Design review of the part built by this model. Coordinates are the model's own, in mm. Face numbers are marked on the shaded views. A direction names the side the tool comes from. Coordinates: 2 decimals unless noted, no trailing zeros. Write each loop counter-clockwise with the first axis right and the second up, starting at its lowest first coordinate (ties: lowest second). Pieces come first, ordered by that corner, then holes.
Q1. Add section C-C, the plane x = -15.5. Give the boundary of the cut face in (y, z), plus the area to 3 significant figures.
Q2. Add section D-D, the plane y = 1.5. Give the boundary of the cut face in (x, z), plus the area to 3 significant figures.
Q3. The part is to be moulded in two halves that separate along X. For the marked faces 4 and 5, say which applies: +X half, -X half, draft (parallel to the pull), parting line (faces both ways), or undercut.
Q4. Clearance check with flat-ended pins moving along their axes: pin 1 Ø0.9 at (y, z) = (10.5, 2) entering from -X; pin 2 Ø1.5 at (y, z) = (-22, -37) entering from -X; pin 3 Ø5 at (x, y) = (-4, -102.5) entering from +Z. State where each tip first meets the part, or that it passes through.
Q5. Add section B-B, the plane y = 15.5. Give the boundary of the cut face in (x, z).
Q6. Machinability: for the marked faces 1, 2 and 3, which of the approach directions +Z, -Z, +X, -X, +Y, -Y give a long, thin tool a straight path to every point of the face, cutting with its end or side? Answer none if there is none.
Q7. To check wall thickness, follow probe 1 along X at (y, z) = (-116.2, -20); probe 2 along X at (y, z) = (-68.5, -9); probe 3 along Y at (x, z) = (-15, 2). State the ranges of each line that lie inside material, in increasing order.
Q8. Add section A-A, the plane z = -35. Give the boundary of the cut face in (x, y), plus the area to 3 significant figures.
Autodesk Inventor part; units mm, degrees
ref_plane "YZ Plane" through (0, 0, 0) normal (1, 0, 0) x (0, 1, 0)
ref_plane "XZ Plane" through (0, 0, 0) normal (0, 1, 0) x (-1, 0, 0)
ref_plane "XY Plane" through (0, 0, 0) normal (0, 0, 1) x (1, 0, 0)
sketch "Boceto1" plane through (0, 0, 0) normal (0, 0, 1) x (1, 0, 0)
  line L0 (-21, 21) -> (21, 21)
  line L1 (21, 21) -> (21, -21)
  line L2 (21, -21) -> (-21, -21)
  line L3 (-21, -21) -> (-21, 21)
  circle A0 centre (0, 0) radius 11.5
  circle A1 centre (-15.5, 15.5) radius 2.25
  circle A2 centre (-15.5, -15.5) radius 2.25
  circle A3 centre (15.5, -15.5) radius 2.25
  circle A4 centre (15.5, 15.5) radius 2.25
  dimension "d0" = 42
  dimension "d1" = 42
  dimension "d2" = 23
  dimension "d6" = 4.5
  dimension "d7" = 4.5
  dimension "d8" = 4.5
  dimension "d9" = 4.5
extrude "Extrusión1" add sketch "Boceto1" along normal blind 3
sketch "Boceto28" plane through (0, 0, 3) normal (0, 0, 1) x (1, 0, 0)
  line L0 (-21.25, -24) -> (21.25, -24)
  line L1 (21.25, -24) -> (21.25, -21)
  line L2 (-21.25, -21) -> (-21.25, -24)
  line L3 (-21, -21) -> (21, -21)
  line L4 (21.25, -21) -> (-21.25, -21)
  point P0 (0, 0)
extrude "Extrusión24" add sketch "Boceto28" against normal blind 43
sketch "Boceto29" plane through (-21.25, -21, -40) normal (0, 1, 0) x (1, 0, 0)
  line L0 (30.25, -12) -> (12.25, -12)
  line L1 (0, 0) -> (42.5, 0)
  line L2 (12.25, 0) -> (30.25, 0)
  line L3 (12.25, 0) -> (12.25, -12)
  line L4 (30.25, 0) -> (30.25, -12)
  point P0 (21.25, -40)
extrude "Extrusión25" cut sketch "Boceto29" against normal blind 3
sketch "Boceto33" plane through (21.25, -24, 3) normal (1, 0, 0) x (0, 0, -1)
  line L0 (43, 0) -> (33, 0)
  line L1 (33, 0) -> (33, 3)
  line L2 (43, 0) -> (46, 0)
  line L3 (46, 0) -> (46, 13)
  line L4 (46, 13) -> (43, 13)
  line L5 (43, 13) -> (33, 3)
  line L6 (0, 45) -> (0, 3)
  line L7 (0, 0) -> (43, 0)
  line L8 (0, 24) -> (0, 0)
  line L9 (0, 0) -> (24, 0)
  line L10 (24, 0) -> (24, 3)
  line L11 (0, 3) -> (43, 3)
  line L12 (0, 24) -> (3, 24)
  line L13 (3, 45) -> (3, 3)
  line L14 (3, 24) -> (24, 3)
  point P0 (0, 3)
  dimension "d153" = 10
  dimension "d154" = 3
  dimension "d155" = 13
  dimension "d156" = 3
  dimension "d181" = 24
extrude "Extrusión28" add sketch "Boceto33" along normal blind 3 contours L0 L1 L5 L4 L3 L2 | L7 L8 L11 L10 | L11 L13 L14 | L11 L6 L12 L13
sketch "Boceto34" plane through (-21.25, -24, 3) normal (-1, 0, 0) x (0, 0, 1)
  line L0 (-46, 0) -> (-46, 13)
  line L1 (-46, 13) -> (-43, 13)
  line L2 (-46, 13) -> (-43, 13)
  line L3 (-43, 13) -> (-33, 3)
  line L4 (-43, 0) -> (-46, 0)
  line L5 (-46, 13) -> (-46, 0)
  line L6 (-46, 0) -> (-33, 0)
  line L7 (-33, 3) -> (-33, 0)
  line L8 (-24, 0) -> (-24, 3)
  line L9 (-24, 3) -> (-3, 24)
  line L10 (0, 24) -> (-3, 24)
  line L11 (-24, 0) -> (0, 0)
  line L12 (0, 0) -> (0, 24)
extrude "Extrusión29" add sketch "Boceto34" along normal blind 3
sketch "Boceto36" plane through (0, 0, -40) normal (0, 0, -1) x (-1, 0, 0)
  line L0 (9, -21) -> (9, -24)
  line L1 (9, -24) -> (21.25, -24)
  line L2 (21.25, -24) -> (21.25, -11)
  line L3 (9, -21) -> (9, -24)
  line L4 (-9, -24) -> (-9, -21)
  line L5 (-9, -21) -> (-9, -24)
  line L6 (-21, -21) -> (-21, 21)
  line L7 (-21.25, -11) -> (-9, -21)
  line L8 (-21.25, -11) -> (-21.25, -24)
  line L9 (24.25, -24) -> (-24.25, -24)
  line L10 (-9, -24) -> (-21.25, -24)
  line L11 (9, -21) -> (21.25, -11)
extrude "Extrusión31" add sketch "Boceto36" along normal blind 3
sketch "Boceto37" plane through (-21, -21, 0) normal (0, 1, 0) x (1, 0, 0)
  line L0 (45.25, 40) -> (45.25, 30)
  line L1 (42.25, 21) -> (42.25, 0)
  line L2 (45.25, 30) -> (42.25, 30)
  line L3 (42.25, 30) -> (42.25, 21)
  line L4 (42.25, 21) -> (45.25, 21)
  line L5 (45.25, 21) -> (45.25, 30)
  line L6 (30, 40) -> (30, 43)
  line L7 (12, 43) -> (12, 28)
  line L8 (30, 40) -> (12, 40)
  line L9 (12, 40) -> (12, 43)
  line L10 (12, 43) -> (30, 43)
  line L11 (30, 43) -> (30, 40)
  line L12 (-0.25, 21) -> (-0.25, 30)
  line L13 (-3.25, 0) -> (-3.25, 21)
  line L14 (-0.25, 30) -> (-3.25, 30)
  line L15 (-3.25, 30) -> (-3.25, 21)
  line L16 (-3.25, 21) -> (-0.25, 21)
  line L17 (-0.25, 21) -> (-0.25, 30)
extrude "Extrusión32" add sketch "Boceto37" against normal blind 3
sketch "Boceto38" plane through (0, 0, 3) normal (0, 0, 1) x (1, 0, 0)
  line L0 (-21.25, 0) -> (-21.25, -21)
  line L1 (-21, -21) -> (-21.25, -21)
  line L2 (-21.25, 0) -> (-21, 0)
  line L3 (-21, 0) -> (-21, -21)
  line L4 (-21, -21) -> (-21.25, -21)
  line L5 (-21.25, -21) -> (-21.25, 0)
  line L6 (21, -21) -> (21, 21)
  line L7 (21.25, 0) -> (21.25, -21)
  line L8 (21, -21) -> (21.25, -21)
  line L9 (21.25, -21) -> (21.25, 0)
  line L10 (21.25, 0) -> (21, 0)
  line L11 (21, 0) -> (21, -21)
extrude "Extrusión33" add sketch "Boceto38" against normal blind 3
sketch "Boceto50" plane through (24.25, -24, -43) normal (0, -1, 0) x (1, 0, 0)
  line L0 (-45.5, 0) -> (-48.5, 0)
  line L1 (-48.5, 0) -> (-48.5, 46)
  line L2 (-48.5, 0) -> (-48.5, 46)
  line L3 (-48.5, 46) -> (-42.5, 46)
  line L4 (-42.5, 46) -> (-42.5, 3)
  line L5 (-48.5, 0) -> (0, 0)
  line L6 (-48.5, 0) -> (0, 0)
  line L7 (0, 0) -> (0, 46)
  line L8 (0, 46) -> (-6, 46)
  line L9 (-6, 46) -> (-6, 3)
  line L10 (-42.5, 3) -> (-6, 3)
  dimension "d183" = 6
  dimension "d184" = 6
extrude "Extrusión39" add sketch "Boceto50" along normal blind 94
sketch "Boceto51" plane through (24.25, -24, 3) normal (1, 0, 0) x (0, 0, -1)
  line L0 (18, -94) -> (28, -94)
  line L1 (28, -94) -> (28, -91)
  line L2 (28, -91) -> (18, -91)
  line L3 (18, -91) -> (18, -94)
  point P0 (3, 24)
  dimension "d171" = 10
  dimension "d172" = 3
extrude "Extrusión40" add sketch "Boceto51" along normal blind 10
sketch "Boceto52" plane through (-24.25, -24, 3) normal (-1, 0, 0) x (0, 0, 1)
  line L0 (0, -94) -> (-46, -94)
  line L1 (-18, -91) -> (-18, -94)
  line L2 (-23, -94) -> (-18, -94)
  line L3 (-18, -94) -> (-18, -91)
  line L4 (-28, -91) -> (-18, -91)
  line L5 (-18, -91) -> (-28, -91)
  line L6 (-28, -94) -> (-28, -91)
  line L7 (-28, -91) -> (-28, -94)
  line L8 (-28, -94) -> (-23, -94)
  point P0 (-3, 24)
extrude "Extrusión41" add sketch "Boceto52" along normal blind 10
sketch "Boceto56" plane through (-24.25, -115, -15) normal (0, 1, 0) x (1, 0, 0)
  line L0 (48.5, 0) -> (58.5, 0)
  line L1 (48.5, 10) -> (58.5, 10)
  line L2 (0, 10) -> (-10, 10)
  line L3 (0, 0) -> (-10, 0)
  line L4 (-10, 0) -> (-10, 10)
  circle A0 centre (-5, 5) radius 2
  circle A1 centre (53.5, 5) radius 2
  point P0 (24.25, -15)
  dimension "d185" = 4
  dimension "d186" = 4
extrude "Extrusión43" cut sketch "Boceto56" against normal blind 3
sketch "Boceto66" plane through (24.25, -24, 3) normal (1, 0, 0) x (0, 0, -1)
  line L0 (3, 24) -> (24, 3)
  circle A0 centre (23, -7) radius 1.6
  dimension "d224" = 3.2
extrude "Extrusión48" cut sketch "Boceto66" against normal blind 10
sketch "Boceto67" plane through (-24.25, -24, 3) normal (-1, 0, 0) x (0, 0, 1)
  line L0 (0, 24) -> (0, -94)
  circle A0 centre (-23, -7) radius 1.6
  point P0 (-3, 24)
  point P1 (-24, 3)
  dimension "d228" = 3.2
extrude "Extrusión50" cut sketch "Boceto67" against normal blind 10
properties part number "Torre Motor Definitiva Pont" material "Plástico ABS"
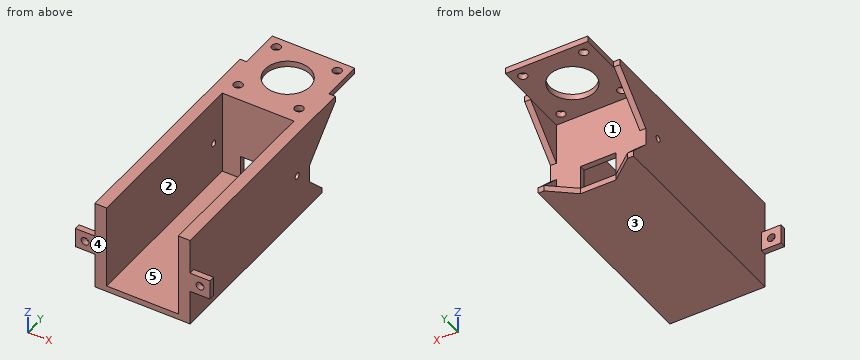
Here are the results:
1. outline: (-118, -43) - (-15.69, -43) - (-15.69, -40) - (-21, -40) - (-21, 0) - (-17.75, 0) - (-17.75, 3) - (-24, 3) - (-24, -40) - (-118, -40) - close; (-13.25, 0) - (13.25, 0) - (13.25, 3) - (-13.25, 3) - close; (17.75, 0) - (21, 0) - (21, 3) - (17.75, 3) - close
1. area: 535 mm2
2. outline: (-21, 0) - (-11.4, 0) - (-11.4, 3) - (-21, 3) - close; (11.4, 0) - (21, 0) - (21, 3) - (11.4, 3) - close
2. area: 57.6 mm2
3. face 4: draft
3. face 5: undercut
4. pin 1: stops at x = -21
4. pin 2: stops at x = -24.25
4. pin 3: stops at z = -40
5. outline: (-21, 0) - (-17.75, 0) - (-17.75, 3) - (-21, 3) - close; (-13.25, 0) - (13.25, 0) - (13.25, 3) - (-13.25, 3) - close; (17.75, 0) - (21, 0) - (21, 3) - (17.75, 3) - close
6. face 1: +Y
6. face 2: +Z, -Y
6. face 3: -Z, +X, -X, +Y, -Y
7. probe 1: x = -34.25 to -31.25, -27.25 to -18.25, 18.25 to 27.25, 31.25 to 34.25
7. probe 2: x = -24.25 to -18.25, 18.25 to 24.25
7. probe 3: y = -24 to -17.69, -13.31 to 13.31, 17.69 to 21
8. outline: (-24.25, -118) - (-18.25, -118) - (-18.25, -24) - (-9, -24) - (-9, -21) - (-21.25, -21) - (-21.25, -16) - (-24.25, -16) - close; (9, -24) - (18.25, -24) - (18.25, -118) - (24.25, -118) - (24.25, -16) - (21.25, -16) - (21.25, -21) - (9, -21) - close
8. area: 1,250 mm2
